The model under review builds one solid part; all positions refer to its coordinate system, in mm. A direction names the side the tool comes from. Give positions to 0.01 mm unless a question says otherwise; leave off trailing zeros. Order: outer loops, then holes, each group sorted by start corner. A loop starts at its lowest first (then second) coordinate and runs counter-clockwise, first axis right, second up.
```python
from build123d import *

# Parameters (mm, degrees)
EXTRUDE_1_DEPTH     = 2
SKETCH_2_R          = 2
SKETCH_2_R_2        = 1.5
SKETCH_2_R_3        = 1
CUT_EXTRUDE_1_DEPTH = 2


with BuildPart() as part:
    # 草图1 → 凸台-拉伸1 (new body)
    with BuildSketch(Plane.XY):
        with BuildLine():
            Line((41.140127792, 10.241950634), (30.684526782, 2.920859991))
            ThreePointArc((30.684526782, 2.920859991), (29.097882601, 2.861150852), (27.763932023, 2))
            Line((27.763932023, 2), (2.236067977, 2))
            ThreePointArc((2.236067977, 2), (-3, 0), (2.236067977, -2))
            Line((2.236067977, -2), (27.763932023, -2))
            ThreePointArc((27.763932023, -2), (30.902117399, -2.861150852), (32.978832528, -0.355748187))
            Line((32.978832528, -0.355748187), (43.434433537, 6.965342457))
            ThreePointArc((43.434433537, 6.965342457), (43.925584753, 9.750799418), (41.140127792, 10.241950634))
        make_face()
    extrude(amount=EXTRUDE_1_DEPTH)

    # 草图2 → 切除-拉伸1 (cut)
    with BuildSketch(Plane.XY.offset(2)):
        Circle(SKETCH_2_R)
        with Locations((30, 0)):
            Circle(SKETCH_2_R_2)
        with Locations((42.287280664, 8.603646545)):
            Circle(SKETCH_2_R_3)
    extrude(amount=-CUT_EXTRUDE_1_DEPTH, mode=Mode.SUBTRACT)


solid = part.part
```
Item 1: Draft analysis for pull direction X (two halves, no side actions). For faces 4 (the flat face through (22.3, 1.8, 0)), 5 (the cylindrical face through (-3, 0, 1)), 6 (the cylindrical face through (43.95, 9.714, 0.986)), state which applies: released by +X, released by -X, zero draft, split by the parting line, or undercut.
Values found:
face 4: zero draft
face 5: undercut
face 6: split by the parting line
Item 2: Take a section at B-B (y = 2.5). Give the boundary of the cut face in (x, z).
Values found:
outline: (-1.66, 0) - (1.66, 0) - (1.66, 2) - (-1.66, 2) - close; (28.34, 0) - (37.06, 0) - (37.06, 2) - (28.34, 2) - close
Item 3: Take a section at A-A (x = 0). Give the boundary of the cut face in (y, z), and give its area (3 significant figures).
Values found:
outline: (-3, 0) - (-2, 0) - (-2, 2) - (-3, 2) - close; (2, 0) - (3, 0) - (3, 2) - (2, 2) - close
area: 4.00 mm2
Item 4: Take a section at D-D (x = 8). Give the boundary of the cut face in (y, z), and give its area (3 significant figures).
Values found:
outline: (-2, 0) - (2, 0) - (2, 2) - (-2, 2) - close
area: 8.00 mm2
Item 5: For line 1 (Y direction, x = 0, z = 1.25); line 2 (X direction, y = 0.25, z = 0.1); line 3 (Y direction, x = 30, z = 0.6), list the stretches that pass through material, from the lowest coordinate up.
Values found:
line 1: y = -3 to -2, 2 to 3
line 2: x = -2.99 to -1.98, 1.98 to 28.52, 31.48 to 33.84
line 3: y = -3 to -1.5, 1.5 to 3
Item 6: For faces 1 (the flat face through (15, 2, 1)), 2 (the flat face through (15, -2, 1)), 3 (the flat face through (38.13, 3.25, 0.99)), list the 3-axis set-ups (+Z, -Z, +X, -X, +Y, -Y) from which the entire face can be reached by the end or side of a thin tool; tool diameter is ignored.
Values found:
face 1: +Z, -Z, +Y
face 2: +Z, -Z, -Y
face 3: +Z, -Z, +X, -Y
Item 7: Take a section at C-C (z = 0.4). Give the boundary of the cut face in (x, y), and give its area (3 significant figures).
Values found:
outline: (2.24, -2) - (27.76, -2) arc R3 ccw to (32.98, -0.36) - (43.43, 6.97) arc R2 ccw to (41.14, 10.24) - (30.68, 2.92) arc R3 ccw to (27.76, 2) - (2.24, 2) arc R3 ccw (long way) to start; hole circle Ø4 at (0, 0); hole circle Ø3 at (30, 0); hole circle Ø2 at (42.29, 8.6)
area: 187 mm2
Item 8: Clearance check with flat-ended pins moving along their axes: pin 1 Ø1 at (x, z) = (8.5, 1.5) entering from +Y; pin 2 Ø1 at (x, z) = (14.5, 1.5) entering from -Y. State where each tip first meets the part, or that it passes through.
Values found:
pin 1: stops at y = 2
pin 2: stops at y = -2
